```python
from build123d import *

# Parameters (mm, degrees)
SKETCH_1_R          = 18.5
SKETCH_1_R_2        = 6
SKETCH_1_R_3        = 1.365103645
EXTRUDE_4_DEPTH     = 19
SKETCH_1_4_R        = 6
EXTRUDE_5_DEPTH     = 6
EXTRUDE_6_DEPTH     = 21
SKETCH_1_6_R        = 1.365103645
CUT_EXTRUDE_2_DEPTH = 6
SKETCH_5_R          = 16.25
EXTRUDE_8_DEPTH     = 23
SKETCH_6_R          = 7.5
EXTRUDE_10_DEPTH    = 10.5


with BuildPart() as part:
    # Sketch 1 → Extrude 4 (new body)
    # profile 1 of 9: a face of its own
    with BuildSketch(Plane(origin=(0, 0, 0), x_dir=(1, 0, 0), z_dir=(0, 1, 0))):
        with Locations(Location((0, 0, 0), (0, 0, 270))):
            Circle(SKETCH_1_R)
        with Locations((0, 7)):
            Circle(SKETCH_1_R_2, mode=Mode.SUBTRACT)
        with Locations((-7.75, -13.423393759)):
            Circle(SKETCH_1_R_3, mode=Mode.SUBTRACT)
        with Locations((7.75, -13.423393759)):
            Circle(SKETCH_1_R_3, mode=Mode.SUBTRACT)
        with Locations((15.5, 0)):
            Circle(SKETCH_1_R_3, mode=Mode.SUBTRACT)
        with Locations((7.75, 13.423393759)):
            Circle(SKETCH_1_R_3, mode=Mode.SUBTRACT)
        with Locations((-7.75, 13.423393759)):
            Circle(SKETCH_1_R_3, mode=Mode.SUBTRACT)
        with Locations((-15.5, 0)):
            Circle(SKETCH_1_R_3, mode=Mode.SUBTRACT)
    # profile 2 of 9: a face of its own
    with BuildSketch(Plane(origin=(0, 0, 0), x_dir=(1, 0, 0), z_dir=(0, 1, 0))):
        with Locations((0, 7)):
            Circle(SKETCH_1_R_2)
        with BuildLine():
            ThreePointArc((-2.236067977, 9), (0, 4), (2.236067977, 9))
            Line((2.236067977, 9), (-2.236067977, 9))
        make_face(mode=Mode.SUBTRACT)
    # profile 3 of 9: a face of its own
    with BuildSketch(Plane(origin=(0, 0, 0), x_dir=(1, 0, 0), z_dir=(0, 1, 0))):
        with BuildLine():
            Line((-2.236067977, 9), (2.236067977, 9))
            ThreePointArc((2.236067977, 9), (0, 4), (-2.236067977, 9))
        make_face()
    # profile 4 of 9: a face of its own
    with BuildSketch(Plane(origin=(0, 0, 0), x_dir=(1, 0, 0), z_dir=(0, 1, 0))):
        with Locations((7.75, -13.423393759)):
            Circle(SKETCH_1_R_3)
    # profile 5 of 9: a face of its own
    with BuildSketch(Plane(origin=(0, 0, 0), x_dir=(1, 0, 0), z_dir=(0, 1, 0))):
        with Locations((-7.75, -13.423393759)):
            Circle(SKETCH_1_R_3)
    # profile 6 of 9: a face of its own
    with BuildSketch(Plane(origin=(0, 0, 0), x_dir=(1, 0, 0), z_dir=(0, 1, 0))):
        with Locations((-15.5, 0)):
            Circle(SKETCH_1_R_3)
    # profile 7 of 9: a face of its own
    with BuildSketch(Plane(origin=(0, 0, 0), x_dir=(1, 0, 0), z_dir=(0, 1, 0))):
        with Locations((-7.75, 13.423393759)):
            Circle(SKETCH_1_R_3)
    # profile 8 of 9: a face of its own
    with BuildSketch(Plane(origin=(0, 0, 0), x_dir=(1, 0, 0), z_dir=(0, 1, 0))):
        with Locations((7.75, 13.423393759)):
            Circle(SKETCH_1_R_3)
    # profile 9 of 9: a face of its own
    with BuildSketch(Plane(origin=(0, 0, 0), x_dir=(1, 0, 0), z_dir=(0, 1, 0))):
        with Locations((15.5, 0)):
            Circle(SKETCH_1_R_3)
    extrude(amount=EXTRUDE_4_DEPTH)

    # Sketch 1_4 → Extrude 5 (add)
    # profile 1 of 2: a face of its own
    with BuildSketch(Plane(origin=(0, 0, 0), x_dir=(1, 0, 0), z_dir=(0, 1, 0))):
        with Locations(Location((0, 7, 0), (0, 0, 270))):
            Circle(SKETCH_1_4_R)
        with BuildLine():
            ThreePointArc((-2.236067977, 9), (0, 4), (2.236067977, 9))
            Line((2.236067977, 9), (-2.236067977, 9))
        make_face(mode=Mode.SUBTRACT)
    # profile 2 of 2: a face of its own
    with BuildSketch(Plane(origin=(0, 0, 0), x_dir=(1, 0, 0), z_dir=(0, 1, 0))):
        with BuildLine():
            Line((-2.236067977, 9), (2.236067977, 9))
            ThreePointArc((2.236067977, 9), (0, 4), (-2.236067977, 9))
        make_face()
    extrude(amount=-EXTRUDE_5_DEPTH)

    # Sketch 1_5 → Extrude 6 (add)
    with BuildSketch(Plane(origin=(0, 0, 0), x_dir=(1, 0, 0), z_dir=(0, 1, 0))):
        with BuildLine():
            Line((-2.236067977, 9), (2.236067977, 9))
            ThreePointArc((2.236067977, 9), (0, 4), (-2.236067977, 9))
        make_face()
    extrude(amount=-EXTRUDE_6_DEPTH)

    # Sketch 1_6 → Cut-Extrude 2 (cut)
    with BuildSketch(Plane(origin=(0, 0, 0), x_dir=(1, 0, 0), z_dir=(0, 1, 0))):
        with Locations(Location((-15.5, 0, 0), (0, 0, 270))):
            Circle(SKETCH_1_6_R)
        with Locations(Location((-7.75, 13.423393759, 0), (0, 0, 270))):
            Circle(SKETCH_1_6_R)
        with Locations(Location((7.75, 13.423393759, 0), (0, 0, 270))):
            Circle(SKETCH_1_6_R)
        with Locations(Location((15.5, 0, 0), (0, 0, 270))):
            Circle(SKETCH_1_6_R)
        with Locations(Location((7.75, -13.423393759, 0), (0, 0, 270))):
            Circle(SKETCH_1_6_R)
        with Locations(Location((-7.75, -13.423393759, 0), (0, 0, 270))):
            Circle(SKETCH_1_6_R)
    extrude(amount=CUT_EXTRUDE_2_DEPTH, mode=Mode.SUBTRACT)

    # Sketch 5 → Extrude 8 (add)
    with BuildSketch(Plane(origin=(0, 19, 0), x_dir=(1, 0, 0), z_dir=(0, 1, 0))):
        with Locations(Location((0, 0, 0), (0, 0, 270))):
            Circle(SKETCH_5_R)
    extrude(amount=EXTRUDE_8_DEPTH)

    # Sketch 6 → Extrude 10 (add)
    with BuildSketch(Plane(origin=(0, 42, 0), x_dir=(1, 0, 0), z_dir=(0, 1, 0))):
        with Locations(Location((0, 0, 0), (0, 0, 90))):
            Circle(SKETCH_6_R)
    extrude(amount=EXTRUDE_10_DEPTH)


solid = part.part
```
Model file for the job. Use its own axes, mm. A direction names the side the tool comes from. Coordinates: 2 decimals unless noted, no trailing zeros. Order: outer loops, then holes, each group sorted by start corner. A loop starts at its lowest first (then second) coordinate and runs counter-clockwise, first axis right, second up. Notation, with made-up numbers: (6, -14.75) -> (33, -14.75) arc R24 ccw to (33, 11.25) -> close; hole circle Ø8 at (64.5, -37.5). An arc over 180 degrees is marked (long way). Return JSON: item names as keys, results as strings.
Item 1: Slice it at A-A (z = 0). Write the cut outline in (x, y), then the cut area to 3 significant figures.
Model answer:
{"outline": "(-18.5, 0) -> (-16.87, 0) -> (-16.87, 6) -> (-14.13, 6) -> (-14.13, 0) -> (14.13, 0) -> (14.13, 6) -> (16.87, 6) -> (16.87, 0) -> (18.5, 0) -> (18.5, 19) -> (16.25, 19) -> (16.25, 42) -> (7.5, 42) -> (7.5, 52.5) -> (-7.5, 52.5) -> (-7.5, 42) -> (-16.25, 42) -> (-16.25, 19) -> (-18.5, 19) -> close", "area": "1,580 mm²"}
Item 2: Slice it at C-C (y = -1.5). Write the cut outline in (x, z).
Model answer:
{"outline": "circle Ø12 at (0, -7)"}
Item 3: Mould opens along X. For faces 4 (the face through (-8.581, 2.958, -14.507)), 5 (the face through (0, -13, -9)), 6 (the face through (-7.086, 9.367, 17.089)) say: pulls with the +X half, pulls with the -X half, needs draft (parallel to the pull), parting line crosses it, or undercut.
Model answer:
{"face 4": "undercut", "face 5": "needs draft", "face 6": "parting line crosses it"}
Item 4: Slice it at D-D (x = -13). Write the cut outline in (y, z).
Model answer:
{"outline": "(0, -13.16) -> (19, -13.16) -> (19, -9.75) -> (42, -9.75) -> (42, 9.75) -> (19, 9.75) -> (19, 13.16) -> (0, 13.16) -> close"}
Item 5: 3-axis set-ups, long thin cutter, end or side, ignore diameter. For faces 1 (the face through (-8, 6, -13)), 2 (the face through (0, -21, -7)), 3 (the face through (-16.4, 19, -0.1)): which of +Z, -Z, +X, -X, +Y, -Y reach the whole face in a straight line?
Model answer:
{"face 1": "-Y", "face 2": "+Z, -Z, +X, -X, -Y", "face 3": "+Y"}
Item 6: Slice it at B-B (x = 0). Write the cut outline in (y, z), then the cut area to 4 significant figures.
Model answer:
{"outline": "(-21, -9) -> (-6, -9) -> (-6, -13) -> (0, -13) -> (0, -18.5) -> (19, -18.5) -> (19, -16.25) -> (42, -16.25) -> (42, -7.5) -> (52.5, -7.5) -> (52.5, 7.5) -> (42, 7.5) -> (42, 16.25) -> (19, 16.25) -> (19, 18.5) -> (0, 18.5) -> (0, -1) -> (-6, -1) -> (-6, -4) -> (-21, -4) -> close", "area": "1,755 mm²"}
Item 7: Wall check: line 1 along X through (y, z) = (4, 0); line 2 along Y through (x, z) = (-13, -4); line 3 along Y through (x, z) = (8, 14.5). Give the ranges that are in metal, low to high. Write a range as from..to.
Model answer:
{"line 1": "x = -18.5..-16.87, -14.13..14.13, 16.87..18.5", "line 2": "y = 0..42", "line 3": "y = 6..19"}
Item 8: Pin check, flat tips, straight feed: P1, Ø10, axis at x = 13, z = -14, coming from the +Y side; P2, Ø5, axis at x = 1.5, z = 2.5, coming from the -Y side; P3, Ø1.5, axis at y = 38.5, z = 3.5, coming from the +X side. Stop position of each tip, or through.
Model answer:
{"P1": "stops at y = 42", "P2": "stops at y = 0", "P3": "stops at x = 16.02"}
